Verification items for this drawing (mm, ordinates from the low corner). Round coordinates to 2 decimals unless told otherwise and drop trailing zeros. Loops run counter-clockwise (first coordinate to the right, second up) from the corner with the lowest first, then second, coordinate; pieces in that order, holes last. Notation, with made-up numbers: (24.5, 15) -> (31.5, 15) arc R19 ccw to (31.5, 30) -> close; hole circle Ø9 at (2, -34). An arc over 180 degrees is marked (long way). One line per question, with ' | ' between items.
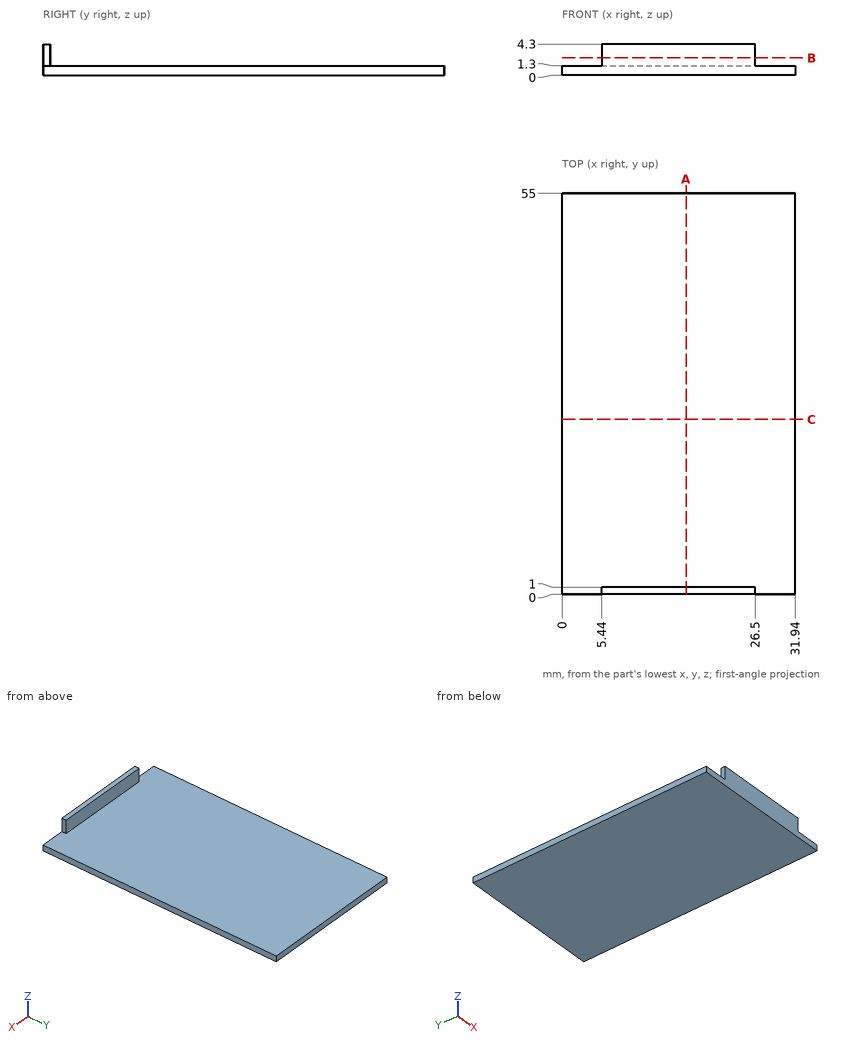
(1) Go/stop test with flat-tipped pins: pin 1 (12 mm diameter, centred on x = 11.5, y = 30.5, fed in from +Z); pin 2 (0.5 mm diameter, centred on y = 0.5, z = 3, fed in from +X). Record where each tip stops, or that it passes through.
Answer:
pin 1: stops at z = 1.3 | pin 2: stops at x = 26.5
(2) Sectioned sample at A-A, the plane x = 17. Record the cut outline in (y, z), and give its area (3 significant figures).
Answer:
outline: (0, 0) -> (55, 0) -> (55, 1.3) -> (1, 1.3) -> (1, 4.3) -> (0, 4.3) -> close | area: 74.5 mm2
(3) Sectioned sample at C-C, the plane y = 24. Record the cut outline in (x, z), and give its area (3 significant figures).
Answer:
outline: (0, 0) -> (31.94, 0) -> (31.94, 1.3) -> (0, 1.3) -> close | area: 41.5 mm2
(4) Sectioned sample at B-B, the plane z = 2.4. Record the cut outline in (x, y).
Answer:
outline: (5.44, 0) -> (26.5, 0) -> (26.5, 1) -> (5.44, 1) -> close
(5) Scan lines: probe 1 along Y at (x, z) = (26, 3.3); probe 2 along Z at (x, y) = (5.5, 51). Record each from-to range of solid material in increasing order.
Answer:
probe 1: y = 0 to 1 | probe 2: z = 0 to 1.3
